Could you check a few things on this model? Use its own coordinates, in mm. A direction names the side the tool comes from. Round coordinates to 2 decimals unless told otherwise and drop trailing zeros. Loops run counter-clockwise (first coordinate to the right, second up) from the corner with the lowest first, then second, coordinate; pieces in that order, holes last. Notation, with made-up numbers: M -15,5 L -11,5 A30 cw -11,30 Z; hole C 1,-27.75 d7. An arc over 180 degrees is marked long. One line per item, written item: value. Start each with the question number.
Q1. Imagine slicing it at D-D (z = 1). Please give me the cut outline in (x, y), then the cut area to 3 significant figures.
Q2. Please list where these lines run through material, in increasing order: line 1 along Z through (x, y) = (23, 0.65); line 2 along Z through (x, y) = (31.25, 0.7); line 3 along X through (y, z) = (1.9, 12.5).
Q3. Which directions (+Z, -Z, +X, -X, +Y, -Y) give clear straight access to the entire face, cutting with the end or side of a thin tool? Please do faces 4 (the face through (27, 0, 1)), 5 (the face through (36, 1, -21.574)).
Q4. Thinking about a two-plate mould opening in X: for faces 1 (the face through (24.18, 1.48, 45.93)), 2 (the face through (29.069, 1, 14)), 3 (the face through (27, 3, 1)), which applies, released by +X, released by -X, zero draft, split by the parting line, or undercut?
Q5. Imagine slicing it at B-B (x = 45.75). Please give me the cut outline in (y, z), then the cut area to 3 significant figures.
Q6. Imagine slicing it at A-A (y = 2.55). Please give me the cut outline in (x, z).
Q7. Imagine slicing it at C-C (z = 47.5). Please give me the cut outline in (x, y).
Q8. I'm going to push flat-ended pins straight in: pin 1 Ø1 at (x, y) = (40.5, 2) entering from +Z; pin 2 Ø8 at (x, z) = (36.5, 27.5) entering from +Y; pin 3 Ø1 at (x, y) = (25, 1) entering from +Z; pin 4 Ø1 at (y, z) = (1.5, 34.5) entering from +X. Where does each tip first touch, or does it pass through?
from build123d import *

# Parameters (mm, degrees)
SKETCH1_R           = 2.5
BOSS_EXTRUDE1_DEPTH = 3


with BuildPart() as part:
    # Sketch1 → Boss-Extrude1 (new body)
    # profile 1 of 4: a face of its own
    with BuildSketch(Plane(origin=(0, 0, 0), x_dir=(1, 0, 0), z_dir=(0, 1, 0))):
        with BuildLine():
            Line((19.068769591, 26.574235382), (19.068769591, -48.425764618))
            ThreePointArc((19.068769591, -48.425764618), (24.068769591, -53.425764618), (29.068769591, -48.425764618))
            Line((29.068769591, -48.425764618), (29.068769591, 21.574235382))
            Line((29.068769591, 21.574235382), (24.068769591, 21.574235382))
            Line((24.068769591, 21.574235382), (24.068769591, 24.074235382))
            ThreePointArc((24.068769591, 24.074235382), (22.301002638, 24.806468429), (21.568769591, 26.574235382))
            Line((21.568769591, 26.574235382), (19.068769591, 26.574235382))
        make_face()
        with Locations(Location((24.068769591, -48.425764618, 0), (0, 0, 270))):
            Circle(SKETCH1_R, mode=Mode.SUBTRACT)
    # profile 2 of 4: a face of its own
    with BuildSketch(Plane(origin=(0, 0, 0), x_dir=(1, 0, 0), z_dir=(0, 1, 0))):
        with BuildLine():
            Line((44.068769591, 31.574235382), (24.068769591, 31.574235382))
            Line((24.068769591, 31.574235382), (24.068769591, 29.074235382))
            ThreePointArc((24.068769591, 29.074235382), (25.836536544, 28.342002335), (26.568769591, 26.574235382))
            Line((26.568769591, 26.574235382), (29.068769591, 26.574235382))
            Line((29.068769591, 26.574235382), (29.068769591, 21.574235382))
            Line((29.068769591, 21.574235382), (44.068769591, 21.574235382))
            ThreePointArc((44.068769591, 21.574235382), (49.068769591, 26.574235382), (44.068769591, 31.574235382))
        make_face()
        with Locations(Location((44.068769591, 26.574235382, 0), (0, 0, 270))):
            Circle(SKETCH1_R, mode=Mode.SUBTRACT)
    # profile 3 of 4: a face of its own
    with BuildSketch(Plane(origin=(0, 0, 0), x_dir=(1, 0, 0), z_dir=(0, 1, 0))):
        with BuildLine():
            Line((24.068769591, 21.574235382), (29.068769591, 21.574235382))
            Line((29.068769591, 21.574235382), (29.068769591, 26.574235382))
            Line((29.068769591, 26.574235382), (26.568769591, 26.574235382))
            ThreePointArc((26.568769591, 26.574235382), (25.836536544, 24.806468429), (24.068769591, 24.074235382))
            Line((24.068769591, 24.074235382), (24.068769591, 21.574235382))
        make_face()
    # profile 4 of 4: a face of its own
    with BuildSketch(Plane(origin=(0, 0, 0), x_dir=(1, 0, 0), z_dir=(0, 1, 0))):
        with BuildLine():
            ThreePointArc((24.068769591, 31.574235382), (20.533235685, 30.109769288), (19.068769591, 26.574235382))
            Line((19.068769591, 26.574235382), (21.568769591, 26.574235382))
            ThreePointArc((21.568769591, 26.574235382), (22.301002638, 28.342002335), (24.068769591, 29.074235382))
            Line((24.068769591, 29.074235382), (24.068769591, 31.574235382))
        make_face()
    extrude(amount=BOSS_EXTRUDE1_DEPTH)


solid = part.part
Report:
1. outline: M 19.07,0 L 29.07,0 L 29.07,3 L 19.07,3 Z
1. area: 30.0 mm²
2. line 1: z = -31.46 to -28.83, -24.31 to 46.17, 50.69 to 53.31
2. line 2: z = -31.57 to -21.57
2. line 3: x = 19.07 to 29.07
3. face 4: +Z, -Z, +X, -X, -Y
3. face 5: +Z, +X, +Y, -Y
4. face 1: undercut
4. face 2: released by +X
4. face 3: zero draft
5. outline: M 0,-31.28 L 3,-31.28 L 3,-28.42 L 0,-28.42 Z; M 0,-24.72 L 3,-24.72 L 3,-21.87 L 0,-21.87 Z
5. area: 17.2 mm²
6. outline: M 19.07,-26.57 A5 ccw 24.07,-31.57 L 44.07,-31.57 A5 ccw 44.07,-21.57 L 29.07,-21.57 L 29.07,48.43 A5 ccw 19.07,48.43 Z; hole C 24.07,-26.57 d5; hole C 24.07,48.43 d5; hole C 44.07,-26.57 d5
7. outline: M 19.07,0 L 21.75,0 L 21.75,3 L 19.07,3 Z; M 26.39,0 L 29.07,0 L 29.07,3 L 26.39,3 Z
8. pin 1: stops at z = -21.57
8. pin 2: passes through
8. pin 3: stops at z = 53.41
8. pin 4: stops at x = 29.07
